The figure shows three views and two pictorial views of one solid part (mm, origin at its lowest corner). Answer the questions. Coordinates: 2 decimals unless noted, no trailing zeros. Write each loop counter-clockwise with the first axis right and the second up, starting at its lowest first coordinate (ties: lowest second). Pieces come first, ordered by that corner, then holes.
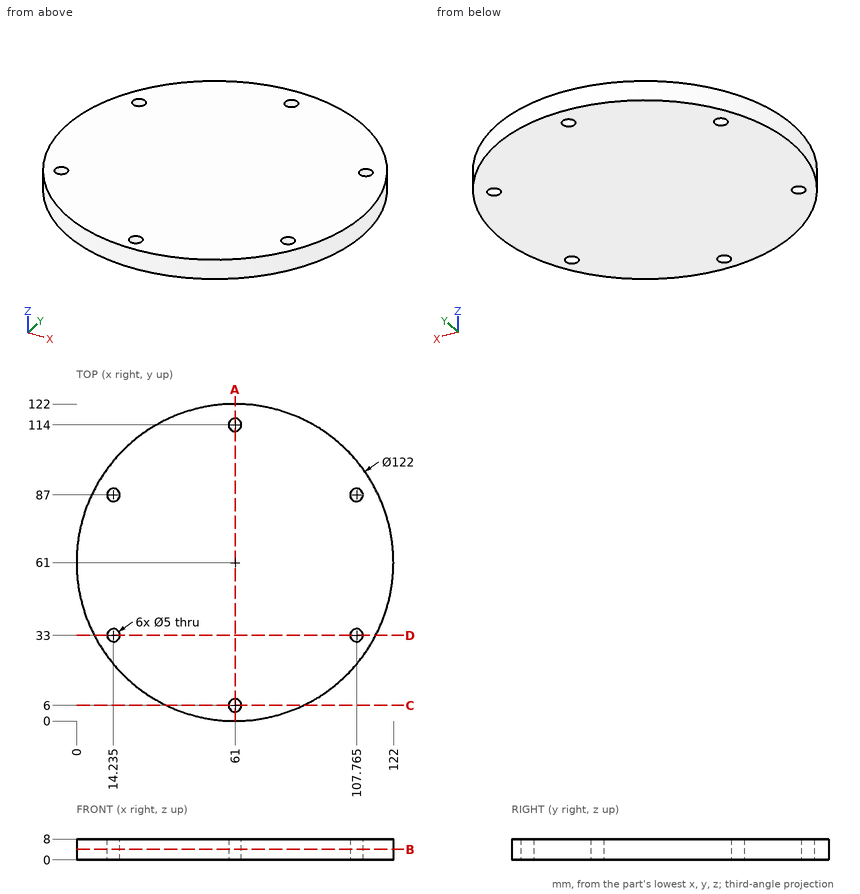
Q1. The part is cut by section A-A, the plane x = 61. Write down the section's boundary in (y, z).
Answers below:
outline: (0, 0) - (3.5, 0) - (3.5, 8) - (0, 8) - close; (8.5, 0) - (111.5, 0) - (111.5, 8) - (8.5, 8) - close; (116.5, 0) - (122, 0) - (122, 8) - (116.5, 8) - close
Q2. The part is cut by section B-B, the plane z = 4. Write down the section's boundary in (x, y) (1 decimal).
Answers below:
outline: circle Ø122 at (61, 61); hole circle Ø5 at (14.2, 33); hole circle Ø5 at (14.2, 87); hole circle Ø5 at (61, 6); hole circle Ø5 at (61, 114); hole circle Ø5 at (107.8, 33); hole circle Ø5 at (107.8, 87)
Q3. The part is cut by section D-D, the plane y = 33. Write down the section's boundary in (x, z) (1 decimal).
Answers below:
outline: (6.8, 0) - (11.7, 0) - (11.7, 8) - (6.8, 8) - close; (16.7, 0) - (105.3, 0) - (105.3, 8) - (16.7, 8) - close; (110.3, 0) - (115.2, 0) - (115.2, 8) - (110.3, 8) - close
Q4. The part is cut by section C-C, the plane y = 6. Write down the section's boundary in (x, z).
Answers below:
outline: (34.62, 0) - (58.5, 0) - (58.5, 8) - (34.62, 8) - close; (63.5, 0) - (87.38, 0) - (87.38, 8) - (63.5, 8) - close
Q5. Find the intervals of material crossed by probe 1 along Y at (x, z) = (61, 4.25); probe 2 along X at (y, z) = (35, 5.25) (1 decimal); probe 3 along X at (y, z) = (87, 2) (1 decimal), in increasing order.
Answers below:
probe 1: y = 0 to 3.5, 8.5 to 111.5, 116.5 to 122
probe 2: x = 5.8 to 12.7, 15.7 to 106.3, 109.3 to 116.2
probe 3: x = 5.8 to 11.7, 16.7 to 105.3, 110.3 to 116.2
Q6. Given pin 1 (4 mm diameter, centred on y = 42.5, z = 6, fed in from -X); pin 2 (4 mm diameter, centred on y = 57, z = 4, fed in from -X); pin 3 (3 mm diameter, centred on x = 30.5, z = 5, fed in from -Y) (1 decimal), each flat-ended and moving along its own axis, determine where each tip first touches the part or whether it passes through.
Answers below:
pin 1: stops at x = 2.27
pin 2: stops at x = 0.03
pin 3: stops at y = 7.3
